from build123d import *

# Parameters (mm, degrees)
BOSS_EXTRUDE1_DEPTH       = 3.9
SKETCH2_R                 = 1
CUT_EXTRUDE3_DEPTH        = 29.385031266
BOSS_EXTRUDE11_DEPTH      = 10
BOSS_EXTRUDE11_DEPTH_BACK = 15
SKETCH161_R               = 8
CUT_EXTRUDE5_DEPTH        = 10


with BuildPart() as part:
    # Sketch1 → Boss-Extrude1 (new body)
    with BuildSketch(Plane.XY):
        Polygon((17.5, 15), (15, 17.5), (-15, 17.5), (-17.5, 15), (-17.5, -15), (-15, -17.5), (15, -17.5), (17.5, -15), align=None)
    extrude(amount=BOSS_EXTRUDE1_DEPTH)

    # Sketch2 → Cut-Extrude3 (cut, through all)
    with BuildSketch(Plane.XY.offset(13.9)):
        with Locations((-13.55, 12.55)):
            Circle(SKETCH2_R)
        with Locations((-13.55, -12.55)):
            Circle(SKETCH2_R)
        with Locations((13.55, 12.55)):
            Circle(SKETCH2_R)
        with Locations((13.55, -12.55)):
            Circle(SKETCH2_R)
    extrude(amount=-CUT_EXTRUDE3_DEPTH, mode=Mode.SUBTRACT)

    # Sketch161 → Boss-Extrude11 (add, two sides: drawn at the far end of the back side and taken through both)
    with BuildSketch(Plane(origin=(0, 3.125608415, -6.702888877), x_dir=(-1, 0, 0), z_dir=(0, 0.42261826174068795, -0.9063077870366554)).offset(-BOSS_EXTRUDE11_DEPTH_BACK)):
        Polygon((-8.5, 11), (-11, 8.5), (-11, -8.5), (-8.5, -11), (8.5, -11), (11, -8.5), (11, 8.5), (8.5, 11), align=None)
        with Locations(Location((0, 0, 0), (0, 0, 270))):
            Circle(SKETCH161_R, mode=Mode.SUBTRACT)
    extrude(amount=BOSS_EXTRUDE11_DEPTH + BOSS_EXTRUDE11_DEPTH_BACK)

    # Sketch162 → Cut-Extrude5 (cut)
    with BuildSketch(Plane.XY.offset(13.9)):
        Polygon((-17.5, 15), (-15, 17.5), (15, 17.5), (17.5, 15), (17.5, -15), (15, -17.5), (-15, -17.5), (-17.5, -15), align=None)
    extrude(amount=-CUT_EXTRUDE5_DEPTH, mode=Mode.SUBTRACT)


solid = part.part
CAD build for the part. Positions are in the model's coordinates, mm. A direction names the side the tool comes from. Round coordinates to 2 decimals unless told otherwise and drop trailing zeros. Order: outer loops, then holes, each group sorted by start corner. A loop starts at its lowest first (then second) coordinate and runs counter-clockwise, first axis right, second up. Notation, with made-up numbers: (-31, -30.5) - (-27, -30.5) arc R10 cw to (-27, -11.5) - close; hole circle Ø11 at (76, 58.5). An arc over 180 degrees is marked (long way). Return JSON: item names as keys, results as strings.
(1) Cut at A-A (x = 13.55). Give the cut face in (y, z).
Answer key:
{"outline": "(-17.5, 0) - (-13.55, 0) - (-13.55, 3.9) - (-17.5, 3.9) - close; (-11.55, 0) - (11.55, 0) - (11.55, 3.9) - (-11.55, 3.9) - close; (13.55, 0) - (17.5, 0) - (17.5, 3.9) - (13.55, 3.9) - close"}
(2) Cut at D-D (x = -6.5). Give the cut face in (y, z) (3 decimals).
Answer key:
{"outline": "(-17.5, 0) - (-12.137, 0) - (-2.618, -20.415) - (3.125, -17.737) - (-5.146, 0) - (5.146, 0) - (11.579, -13.795) - (17.321, -11.117) - (12.137, 0) - (17.5, 0) - (17.5, 3.9) - (-17.5, 3.9) - close"}
(3) Cut at C-C (y = -11). Give the cut face in (x, z).
Answer key:
{"outline": "(-17.5, 0) - (-9.53, 0) - (-8.5, -2.44) - (8.5, -2.44) - (9.53, 0) - (17.5, 0) - (17.5, 3.9) - (-17.5, 3.9) - close"}
(4) Pull direction Z, two halves, no side cores. Call faces 3 (the face through (-11, 4, -8)), 4 (the face through (-9.77, 13.29, -5.48)), 5 (the face through (9.768, -6.295, -9.529)), 6 (the face through (-0.1, 14.7, -5.5)): +Z half, -Z half, draft (parallel to the pull), parting line (faces both ways), or undercut.
Answer key:
{"face 3": "draft", "face 4": "undercut", "face 5": "-Z half", "face 6": "undercut"}
(5) Tool access for faces 1 (the face through (14.504, -12.25, 1.977)), 2 (the face through (11, 4, -8)): list every direction of +Z, -Z, +X, -X, +Y, -Y with a clear straight run to the whole face (end or side of a thin tool).
Answer key:
{"face 1": "+Z, -Z", "face 2": "-Z, +X, +Y, -Y"}
(6) Wall check: probe 1 along Y at (x, z) = (13.55, 2.2); probe 2 along Z at (x, y) = (-2, 1); probe 3 along Z at (x, y) = (-3, -4). Give the ranges that are in metal, low to high. Write a range as from..to.
Answer key:
{"probe 1": "y = -17.5..-13.55, -11.55..11.55, 13.55..17.5", "probe 2": "z = 0..3.9", "probe 3": "z = -17.45..-8.97, 0..3.9"}
(7) Cut at B-B (z = 1.25). Give the cut face in (x, y), then the cut area to 3 significant figures.
Answer key:
{"outline": "(-17.5, -15) - (-15, -17.5) - (15, -17.5) - (17.5, -15) - (17.5, 15) - (15, 17.5) - (-15, 17.5) - (-17.5, 15) - close; hole circle Ø2 at (-13.55, -12.55); hole circle Ø2 at (-13.55, 12.55); hole circle Ø2 at (13.55, -12.55); hole circle Ø2 at (13.55, 12.55)", "area": "1,200 mm^2"}
(8) Pin check, flat tips, straight feed: pin 1 Ø1.8 at (x, y) = (-13.55, 12.55) entering from +Z; pin 2 Ø4 at (y, z) = (8, -8.5) entering from -X; pin 3 Ø4 at (x, z) = (-11, -9) entering from -Y; pin 4 Ø8 at (x, y) = (2.5, 2) entering from -Z. Stop position of each tip, or through.
Answer key:
{"pin 1": "passes through", "pin 2": "stops at x = -11", "pin 3": "stops at y = -7.58", "pin 4": "stops at z = -20.13"}
